Read the model definition and answer for the solid it produces. Units are mm, in the model's axes. A direction names the side the tool comes from. Round coordinates to 2 decimals unless told otherwise and drop trailing zeros. Write each loop counter-clockwise with the first axis right and the second up, starting at its lowest first coordinate (ties: lowest second). Pieces come first, ordered by that corner, then holes. Notation, with made-up numbers: (22.5, -11) -> (53.5, -11) arc R24 ccw to (53.5, 15) -> close; hole circle Ø5 at (37.5, 15.25). An arc over 180 degrees is marked (long way). Return JSON: item names as keys, results as strings.
from build123d import *

# Parameters (mm, degrees)
CHAMFER1_SIZE      = 0.5
SKETCH2_R          = 1
CUT_EXTRUDE1_DEPTH = 27.420872431


with BuildPart() as part:
    # Sketch1 → Revolve1 (revolve)
    with BuildSketch(Plane.XY, mode=Mode.PRIVATE) as revolve1_sk:
        Polygon((0, 15.75), (-15, 15.75), (-15, 8.05), (-7.5, 8.05), (-7.5, 0), (-2.5, 0), (-2.5, 10), (0, 10), align=None)
    revolve(revolve1_sk.sketch.rotate(Axis((0, 0, 0), (0, 1, 0)), 270), axis=Axis((0, 0, 0), (0, 1, 0)))

    # Chamfer1
    chamfer1_edges = [part.edges().sort_by_distance(p)[0] for p in [
        (0, 0, 7.5),
        (0, 8.05, 7.5),
        (0, 8.05, 15),
        (0, 15.75, 15),
    ]]
    chamfer(chamfer1_edges, length=CHAMFER1_SIZE)

    # Sketch2 → Cut-Extrude1 (cut, through all)
    with BuildSketch(Plane.XY):
        with Locations(Location((0, 4.5, 0), (0, 0, 90))):
            Circle(SKETCH2_R)
    extrude(amount=-CUT_EXTRUDE1_DEPTH, mode=Mode.SUBTRACT)


solid = part.part
Item 1: Straight lines are drawn through the part: L1, parallel to X at y = 3.5, z = 0; L2, parallel to Y at x = -8.5, z = -11; L3, parallel to X at y = 9.25, z = -0.5. For each, find the intervals that lie inside material, in ascending order. Write a range as [from, to].
Worked answers:
{"L1": "x = [-7.5, -2.5], [2.5, 7.5]", "L2": "y = [8.05, 15.75]", "L3": "x = [-14.99, -2.45], [2.45, 14.99]"}
Item 2: Section B-B (y = 6.5) is taken. Give the vertices of the cut face in (x, z), then the cut area to 3 significant figures.
Worked answers:
{"outline": "circle Ø15 at (0, 0); hole circle Ø5 at (0, 0)", "area": "157 mm2"}
Item 3: Section A-A (x = 0) is taken. Give the vertices of the cut face in (y, z).
Worked answers:
{"outline": "(0, -7) -> (0.5, -7.5) -> (3.5, -7.5) -> (3.5, -2.5) -> (0, -2.5) -> close; (0, 2.5) -> (10, 2.5) -> (10, -2.5) -> (5.5, -2.5) -> (5.5, -7.5) -> (7.55, -7.5) -> (8.05, -8) -> (8.05, -14.5) -> (8.55, -15) -> (15.25, -15) -> (15.75, -14.5) -> (15.75, 14.5) -> (15.25, 15) -> (8.55, 15) -> (8.05, 14.5) -> (8.05, 8) -> (7.55, 7.5) -> (0.5, 7.5) -> (0, 7) -> close"}
Item 4: A tool of negligible diameter and unlimited length cuts with its end or side. For faces 1 (the flat face through (0, 10, 0)), 2 (the flat face through (0, 15.75, 0)), from which of +Z, -Z, +X, -X, +Y, -Y can it reach the whole face along a straight path? Write none if from no direction.
Worked answers:
{"face 1": "-Y", "face 2": "+Z, -Z, +X, -X, +Y"}
Item 5: Section C-C (z = 0) is taken. Give the vertices of the cut face in (x, y), then the cut area to 3 significant figures.
Worked answers:
{"outline": "(-15, 8.55) -> (-14.5, 8.05) -> (-8, 8.05) -> (-7.5, 7.55) -> (-7.5, 0.5) -> (-7, 0) -> (-2.5, 0) -> (-2.5, 10) -> (2.5, 10) -> (2.5, 0) -> (7, 0) -> (7.5, 0.5) -> (7.5, 7.55) -> (8, 8.05) -> (14.5, 8.05) -> (15, 8.55) -> (15, 15.25) -> (14.5, 15.75) -> (-14.5, 15.75) -> (-15, 15.25) -> close", "area": "301 mm2"}
Item 6: For a pull along X with two mould halves and no side action, classify faces 3 (the flat face through (6, 8.05, -6)), 4 (the cylindrical face through (0.6, 3.7, -4.9)), 5 (the cylindrical face through (-0.66, 11.853, 14.985)) as released by +X, released by -X, zero draft, split by the parting line, or undercut.
Worked answers:
{"face 3": "zero draft", "face 4": "undercut", "face 5": "split by the parting line"}
Item 7: Section D-D (y = 11.5) is taken. Give the vertices of the cut face in (x, z).
Worked answers:
{"outline": "circle Ø30 at (0, 0)"}
Item 8: Flat-ended cylindrical pins translate along their axes: pin 1 (1 mm diameter, centred on y = 4.5, z = 9, fed in from +X); pin 2 (5 mm diameter, centred on x = -2.5, y = 4, fed in from -Z); pin 3 (4 mm diameter, centred on y = 12, z = -7.5, fed in from +X); pin 4 (4 mm diameter, centred on y = 9.5, z = -6, fed in from -X). Find the tip coordinate at first contact, or state that the pin passes through.
Worked answers:
{"pin 1": "passes through", "pin 2": "stops at z = -7.5", "pin 3": "stops at x = 13.96", "pin 4": "stops at x = -14.46"}
